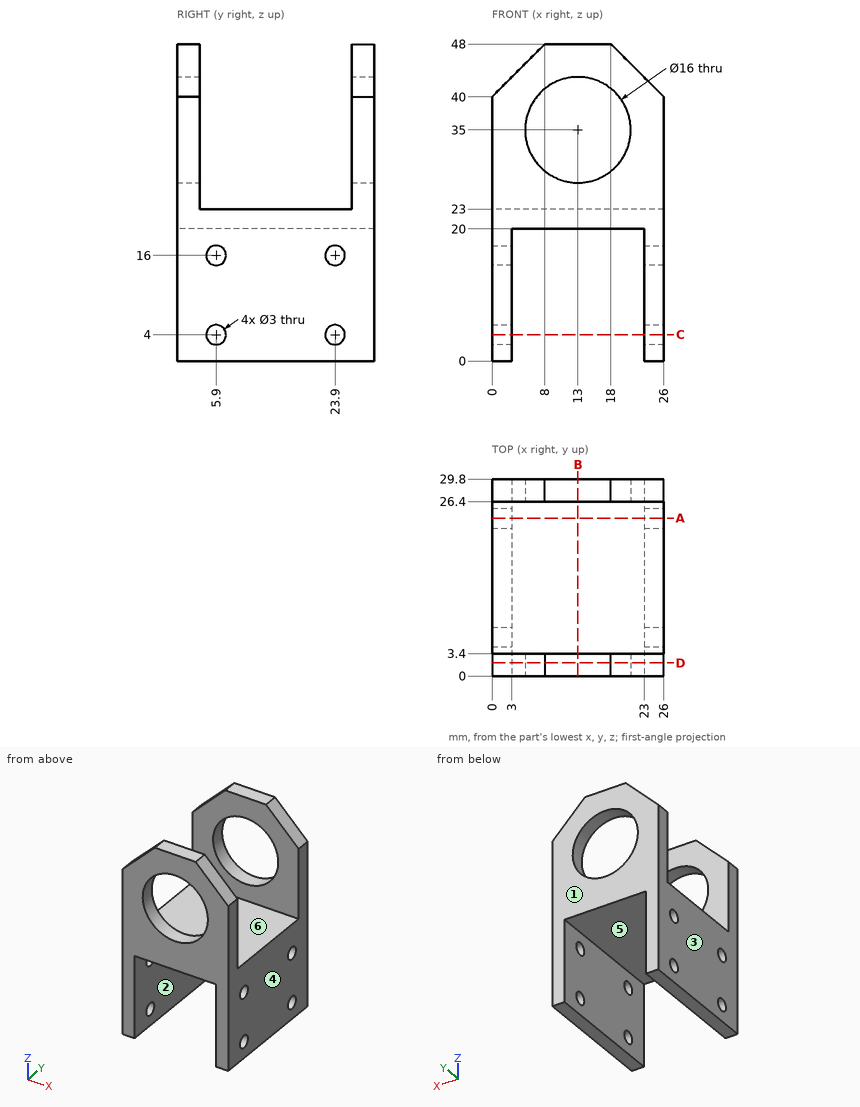
The figure shows three views and two pictorial views of one solid part (mm, origin at its lowest corner). Answer the questions. A direction names the side the tool comes from. Coordinates: 2 decimals unless noted, no trailing zeros. Write each loop counter-clockwise with the first axis right and the second up, starting at its lowest first coordinate (ties: lowest second). Pieces come first, ordered by that corner, then holes. Notation, with made-up numbers: (76, -6.75) -> (90, -6.75) arc R21 cw to (90, 24.25) -> close; hole circle Ø7 at (-8.75, 59). An arc over 180 degrees is marked (long way). Return JSON: item names as keys, results as strings.
1. A tool of negligible diameter and unlimited length cuts with its end or side. For the marked faces 4, 5 and 6, from which of +Z, -Z, +X, -X, +Y, -Y can it reach the whole face along a straight path? Write none if from no direction.
Found:
{"face 4": "+Z, -Z, +X, +Y, -Y", "face 5": "-Z, +Y, -Y", "face 6": "+Z, +X, -X"}
2. A cutting plane is placed at B-B (x = 13). Determine the outline of the cut face in (y, z), and give its area (3 significant figures).
Found:
{"outline": "(0, 20) -> (29.8, 20) -> (29.8, 27) -> (26.4, 27) -> (26.4, 23) -> (3.4, 23) -> (3.4, 27) -> (0, 27) -> close; (0, 43) -> (3.4, 43) -> (3.4, 48) -> (0, 48) -> close; (26.4, 43) -> (29.8, 43) -> (29.8, 48) -> (26.4, 48) -> close", "area": "151 mm2"}
3. Each of these flat-tipped pins is pushed along its axis until it touches: P1, Ø4, axis at y = 5.9, z = 16, coming from the -X side; P2, Ø2.5, axis at y = 5.9, z = 4, coming from the -X side; P3, Ø4, axis at x = 22.5, y = 6.5, coming from the +Z side; P4, Ø6, axis at x = 14, y = 15.5, coming from the -Z side. Where does it stop, or does it pass through?
Found:
{"P1": "x = 0", "P2": "through", "P3": "z = 23", "P4": "z = 20"}
4. A cutting plane is placed at A-A (y = 23.9). Determine the outline of the cut face in (x, z), and give its area (3 significant figures).
Found:
{"outline": "(0, 0) -> (3, 0) -> (3, 2.5) -> (0, 2.5) -> close; (0, 5.5) -> (3, 5.5) -> (3, 14.5) -> (0, 14.5) -> close; (0, 17.5) -> (3, 17.5) -> (3, 20) -> (23, 20) -> (23, 17.5) -> (26, 17.5) -> (26, 23) -> (0, 23) -> close; (23, 0) -> (26, 0) -> (26, 2.5) -> (23, 2.5) -> close; (23, 5.5) -> (26, 5.5) -> (26, 14.5) -> (23, 14.5) -> close", "area": "162 mm2"}
5. Determine the mould class of the marked faces 1, 2 and 3 for opening direction X: pulls with the +X half, pulls with the -X half, needs draft (parallel to the pull), parting line crosses it, or undercut.
Found:
{"face 1": "needs draft", "face 2": "undercut", "face 3": "pulls with the -X half"}
6. A cutting plane is placed at C-C (z = 4). Determine the outline of the cut face in (x, y), and give its area (3 significant figures).
Found:
{"outline": "(0, 0) -> (3, 0) -> (3, 4.4) -> (0, 4.4) -> close; (0, 7.4) -> (3, 7.4) -> (3, 22.4) -> (0, 22.4) -> close; (0, 25.4) -> (3, 25.4) -> (3, 29.8) -> (0, 29.8) -> close; (23, 0) -> (26, 0) -> (26, 4.4) -> (23, 4.4) -> close; (23, 7.4) -> (26, 7.4) -> (26, 22.4) -> (23, 22.4) -> close; (23, 25.4) -> (26, 25.4) -> (26, 29.8) -> (23, 29.8) -> close", "area": "143 mm2"}
7. A cutting plane is placed at D-D (y = 2). Determine the outline of the cut face in (x, z).
Found:
{"outline": "(0, 0) -> (3, 0) -> (3, 20) -> (23, 20) -> (23, 0) -> (26, 0) -> (26, 40) -> (18, 48) -> (8, 48) -> (0, 40) -> close; hole circle Ø16 at (13, 35)"}
8. Find the intervals of material crossed by line 1 along Y through (x, z) = (1.5, 16); line 2 along X through (y, z) = (8.75, 10); line 3 along Y through (x, z) = (2.75, 30), in increasing order. Write a range as from..to.
Found:
{"line 1": "0..4.4, 7.4..22.4, 25.4..29.8", "line 2": "0..3, 23..26", "line 3": "0..3.4, 26.4..29.8"}
